The listing builds one solid part. Answer for the finished solid, in the listing's coordinates (mm). Round coordinates to 2 decimals unless told otherwise and drop trailing zeros. Loops run counter-clockwise (first coordinate to the right, second up) from the corner with the lowest first, then second, coordinate; pieces in that order, holes last. Notation, with made-up numbers: (56.5, 68.5) -> (67.5, 68.5) arc R34 ccw to (67.5, 101.5) -> close; hole circle Ø4 at (69, -27). An arc over 180 degrees is marked (long way). Use a Markdown table: item, result. Add a question column.
Q1. Consider line 1 (X direction, y = 51, z = -0.85); line 2 (Y direction, x = -36.83, z = -2.5) (3 decimals); line 3 (Y direction, x = -133.35, z = -1.65) (3 decimals). Determine where each line is inside the solid, lowest interval first.
Q2. Section A-A on x = -133.35 is taken. Give the vertices of the cut face in (y, z) (3 decimals), then the cut area to 3 significant figures.
Q3. Section B-B on x = -57.15 is taken. Give the vertices of the cut face in (y, z) (3 decimals), then the cut area to 3 significant figures.
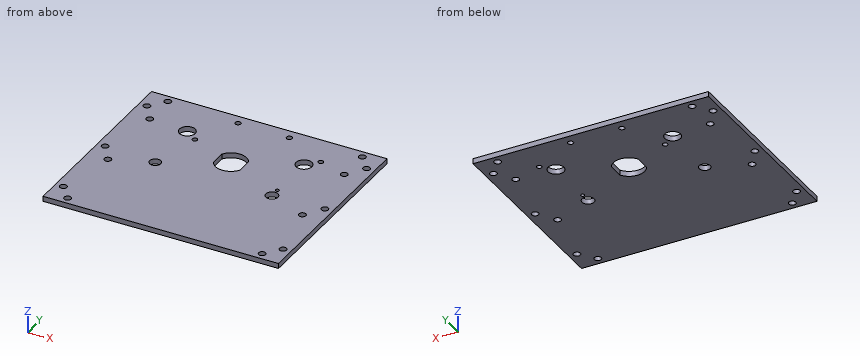
from build123d import *

# Parameters (mm, degrees)
SKETCH1_W                = 146.05
SKETCH1_H                = 123.825
BOSS_EXTRUDE1_DEPTH      = 3.175
F_6_CLEARANCE_HOLE1_D    = 4.3053
SKETCH4_R                = 4.9022
SKETCH4_R_2              = 3.7703125
SKETCH4_R_3              = 3.429
SKETCH4_R_4              = 1.125
SKETCH4_R_5              = 1.5875
SWITCH_MOUNT_HOLES_DEPTH = 4.175
F_4_CLEARANCE_HOLE1_D    = 3.4544


with BuildPart() as part:
    # Sketch1 → Boss-Extrude1 (new body)
    with BuildSketch(Plane.XY):
        with Locations((-73.025, 61.9125)):
            Rectangle(SKETCH1_W, SKETCH1_H)
    extrude(amount=-BOSS_EXTRUDE1_DEPTH)

    # #6 Clearance Hole1 (through all)
    with Locations(Plane(origin=(0, 0, -3.175), x_dir=(-1, 0, 0), z_dir=(0, 0, -1))):
        with Locations((12.7, 119.0625), (133.35, 119.0625), (141.1605, 109.5375), (133.35, 98.425), (141.1605, 61.9125), (133.35, 50.673), (133.35, 4.7625), (12.7, 4.7625), (12.7, 50.673), (12.7, 98.425), (4.8895, 109.5375), (141.1605, 14.2875), (4.8895, 14.2875), (4.8895, 61.9125)):
            Hole(F_6_CLEARANCE_HOLE1_D / 2)

    # Sketch4 → Switch Mount Holes (cut, through all)
    with BuildSketch(Plane(origin=(0, 0, -3.175), x_dir=(-1, 0, 0), z_dir=(0, 0, -1))):
        with Locations((36.83, 96.901)):
            Circle(SKETCH4_R)
        with Locations((36.83, 60.325)):
            Circle(SKETCH4_R_2)
        with Locations((109.22, 60.325)):
            Circle(SKETCH4_R_3)
        with Locations((109.22, 96.901)):
            Circle(SKETCH4_R)
        with Locations((36.830000027, 66.525)):
            Circle(SKETCH4_R_4)
        with Locations((101.514113129, 91.302345472)):
            Circle(SKETCH4_R_5)
        with Locations((30.094807909, 103.636192091)):
            Circle(SKETCH4_R_5)
        with BuildLine():
            Line((81.3435, 85.032269324), (81.3435, 75.241730676))
            ThreePointArc((81.3435, 75.241730676), (73.025, 70.485), (64.7065, 75.241730676))
            Line((64.7065, 75.241730676), (64.7065, 85.032269324))
            ThreePointArc((64.7065, 85.032269324), (73.025, 89.789), (81.3435, 85.032269324))
        make_face()
    extrude(amount=-SWITCH_MOUNT_HOLES_DEPTH, mode=Mode.SUBTRACT)

    # #4 Clearance Hole1 (through all)
    with Locations(Plane.XY):
        with Locations((-88.9, 117.475), (-57.15, 117.475)):
            Hole(F_4_CLEARANCE_HOLE1_D / 2)


solid = part.part
Checked values:
| question | item | result |
|---|---|---|
| 1 | line 1 | x = -146.05 to -135.48, -131.22 to -14.83, -10.57 to 0 |
| 1 | line 2 | y = 0 to 56.555, 64.095 to 65.4, 67.65 to 91.999, 101.803 to 123.825 |
| 1 | line 3 | y = 0 to 2.61, 6.915 to 48.52, 52.826 to 96.272, 100.578 to 116.91, 121.215 to 123.825 |
| 2 | outline | (0, -3.175) -> (2.61, -3.175) -> (2.61, 0) -> (0, 0) -> close; (6.915, -3.175) -> (48.52, -3.175) -> (48.52, 0) -> (6.915, 0) -> close; (52.826, -3.175) -> (96.272, -3.175) -> (96.272, 0) -> (52.826, 0) -> close; (100.578, -3.175) -> (116.91, -3.175) -> (116.91, 0) -> (100.578, 0) -> close; (121.215, -3.175) -> (123.825, -3.175) -> (123.825, 0) -> (121.215, 0) -> close |
| 2 | area | 338 mm2 |
| 3 | outline | (0, -3.175) -> (115.748, -3.175) -> (115.748, 0) -> (0, 0) -> close; (119.202, -3.175) -> (123.825, -3.175) -> (123.825, 0) -> (119.202, 0) -> close |
| 3 | area | 382 mm2 |
